Geometry: final body of the model. Coordinates: model frame, mm. Face numbers are marked on the shaded views. A direction names the side the tool comes from. Coordinates: 2 decimals unless noted, no trailing zeros. Write each loop counter-clockwise with the first axis right and the second up, starting at its lowest first coordinate (ties: lowest second). Pieces come first, ordered by that corner, then holes. Notation, with made-up numbers: (64, -5.5) -> (68, -5.5) arc R13 cw to (68, 1.5) -> close; hole circle Ø1 at (87, 82). An arc over 180 degrees is marked (long way). Answer as a JSON object with one key per item and string values. Group by question number.
```python
from build123d import *

# Parameters (mm, degrees)
SKETCH1_W           = 60
SKETCH1_H           = 30
BOSS_EXTRUDE1_DEPTH = 10
FILLET1_R           = 10
FILLET3_R           = 10
FILLET4_R           = 10
CUT_EXTRUDE1_DEPTH  = 4
CUT_EXTRUDE2_DEPTH  = 4
SKETCH8_R           = 1.5
CUT_EXTRUDE3_DEPTH  = 4
SHELL5_START        = 2
SHELL5_DEPTH        = 8
CUT_EXTRUDE4_DEPTH  = 2
SKETCH11_W          = 6.86286456
SKETCH11_H          = 3.5
BOSS_EXTRUDE2_DEPTH = 1
CUT_EXTRUDE5_DEPTH  = 0.1


# Read off the part's stored shape, not the designer's step: Shell5
with BuildPart() as part:
    # Sketch1 → Boss-Extrude1 (new body)
    with BuildSketch(Plane(origin=(0, 0, 0), x_dir=(1, 0, 0), z_dir=(0, 1, 0))):
        with Locations((-2.582747066, 7.592753862)):
            Rectangle(SKETCH1_W, SKETCH1_H)
    extrude(amount=BOSS_EXTRUDE1_DEPTH)

    # Fillet1
    fillet1_edges = [part.edges().sort_by_distance(p)[0] for p in [
        (27.417252934, 5, 7.407246138),
    ]]
    fillet(fillet1_edges, radius=FILLET1_R)

    # Fillet3
    fillet3_edges = [part.edges().sort_by_distance(p)[0] for p in [
        (-32.582747066, 5, 7.407246138),
    ]]
    fillet(fillet3_edges, radius=FILLET3_R)

    # Fillet4
    fillet4_edges = [part.edges().sort_by_distance(p)[0] for p in [
        (-32.582747066, 5, -22.592753862),
    ]]
    fillet(fillet4_edges, radius=FILLET4_R)

    # Sketch6 → Cut-Extrude1 (cut)
    with BuildSketch(Plane(origin=(0, 10, 0), x_dir=(1, 0, 0), z_dir=(0, 1, 0))):
        Polygon((17.417252934, 22.592753862), (27.417252934, 12.592753862), (27.417252934, 22.592753862), align=None)
    extrude(amount=-CUT_EXTRUDE1_DEPTH, mode=Mode.SUBTRACT)

    # Sketch7 → Cut-Extrude2 (cut)
    with BuildSketch(Plane.XZ):
        Polygon((27.417252934, -22.592753862), (27.417252934, -12.592753862), (17.417252934, -22.592753862), align=None)
    extrude(amount=-CUT_EXTRUDE2_DEPTH, mode=Mode.SUBTRACT)

    # Sketch8 → Cut-Extrude3 (cut)
    with BuildSketch(Plane(origin=(0, 6, 0), x_dir=(1, 0, 0), z_dir=(0, 1, 0))):
        with Locations(Location((24.917252934, 20.092753862, 0), (0, 0, 270))):
            Circle(SKETCH8_R)
    extrude(amount=-CUT_EXTRUDE3_DEPTH, mode=Mode.SUBTRACT)

    # Shell5 outline → Shell5 (cut)
    with BuildSketch(Plane(origin=(0, 0, 0), x_dir=(1, 0, 0), z_dir=(0, 1, 0)).offset(SHELL5_START)):
        with BuildLine():
            Line((25.417252934, 2.592753862), (25.417252934, 11.764326737))
            Line((25.417252934, 11.764326737), (16.588825809, 20.592753862))
            Line((16.588825809, 20.592753862), (-22.582747066, 20.592753862))
            ThreePointArc((-22.582747066, 20.592753862), (-28.239601315, 18.249608111), (-30.582747066, 12.592753862))
            Line((-30.582747066, 12.592753862), (-30.582747066, 2.592753862))
            ThreePointArc((-30.582747066, 2.592753862), (-28.239601315, -3.064100388), (-22.582747066, -5.407246138))
            Line((-22.582747066, -5.407246138), (17.417252934, -5.407246138))
            ThreePointArc((17.417252934, -5.407246138), (23.074107184, -3.064100387), (25.417252934, 2.592753862))
        make_face()
    extrude(amount=SHELL5_DEPTH, mode=Mode.SUBTRACT)

    # Sketch10 → Cut-Extrude4 (cut)
    with BuildSketch(Plane(origin=(0, 0, -22.592753862), x_dir=(-1, 0, 0), z_dir=(0, 0, -1))):
        Polygon((2.582747066, 5.925), (6.032747066, 5.925), (6.032747066, 4.825), (5.282747066, 4.075), (2.582747066, 4.075), (-0.117252934, 4.075), (-0.867252934, 4.825), (-0.867252934, 5.925), align=None)
    extrude(amount=-CUT_EXTRUDE4_DEPTH, mode=Mode.SUBTRACT)

    # Sketch11 → Boss-Extrude2 (add)
    with BuildSketch(Plane(origin=(0, 0, -22.592753862), x_dir=(-1, 0, 0), z_dir=(0, 0, -1))):
        with Locations((12.582747066, 5)):
            Rectangle(SKETCH11_W, SKETCH11_H)
    extrude(amount=BOSS_EXTRUDE2_DEPTH)

    # Sketch12 → Cut-Extrude5 (cut)
    with BuildSketch(Plane(origin=(0, 0, -23.592753862), x_dir=(-1, 0, 0), z_dir=(0, 0, -1))):
        Polygon((12.582747066, 5), (12.735825542, 5), (12.735825542, 6.297110067), (12.428698836, 6.297110067), (12.428698836, 5), align=None)
        with BuildLine():
            Line((12.111519237, 5.882859707), (12.204075045, 5.709453579))
            ThreePointArc((12.204075045, 5.709453579), (12.582747066, 4.195812907), (12.961419087, 5.709453579))
            Line((12.961419087, 5.709453579), (13.053974895, 5.882859707))
            ThreePointArc((13.053974895, 5.882859707), (12.582747066, 3.999251816), (12.111519237, 5.882859707))
        make_face()
    extrude(amount=-CUT_EXTRUDE5_DEPTH, mode=Mode.SUBTRACT)


solid = part.part
```
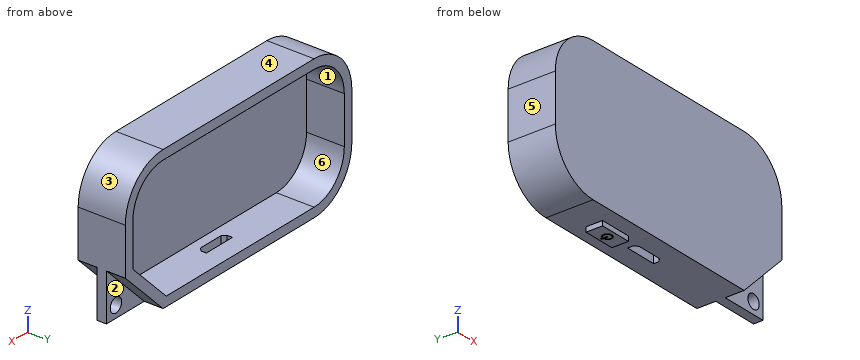
Item 1: Section A-A on y = 8.5. Output: boundary loops of the cut face in (x, z), then the cut area to 3 significant figures.
Item 2: Mould query, pull axis Z, two halves, no side actions, for the marked faces 4, 5 and 6. Classes: +Z half, -Z half, draft (parallel to the pull), parting line (faces both ways), or undercut.
Item 3: Contact query for flat-ended pins moving along their axis: pin 1 (2 mm diameter, centred on x = 7, y = 3, fed in from -Z); pin 2 (4 mm diameter, centred on x = 24.92, z = -20.09, fed in from -Y). Output: stop coordinate, or through.
Item 4: Section B-B on x = -15. Output: boundary loops of the cut face in (y, z), then the cut area to 3 significant figures.
Item 5: Section C-C on z = -20. Output: boundary loops of the cut face in (x, y).
Item 6: Ray query, L1, parallel to Z at x = -2.5, y = 4; L2, parallel to X at y = 5.75, z = -8; L3, parallel to Z at x = -11.5, y = 4.5. Return the intervals inside material, ascending. Write a range as [from, to].
Item 7: Set-up query: the marked faces 1, 2 and 3. Return all of +Z, -Z, +X, -X, +Y, -Y with unobstructed straight access to the full face (end or side cutting, diameter ignored); none if empty.
Item 8: Section D-D on y = 0.75. Output: boundary loops of the cut face in (x, z), then the cut area to 3 significant figures.
Answer sheet:
{
 "1": {"outline": "(-32.58, -12.59) arc R10 ccw to (-22.58, -22.59) -> (17.42, -22.59) -> (27.42, -12.59) -> (27.42, -2.59) arc R10 ccw to (17.42, 7.41) -> (-22.58, 7.41) arc R10 ccw to (-32.58, -2.59) -> close; hole (-30.58, -12.59) arc R8 ccw to (-22.58, -20.59) -> (16.59, -20.59) -> (25.42, -11.76) -> (25.42, -2.59) arc R8 ccw to (17.42, 5.41) -> (-22.58, 5.41) arc R8 ccw to (-30.58, -2.59) -> close", "area": "310 mm^2"},
 "2": {"face 4": "+Z half", "face 5": "draft", "face 6": "undercut"},
 "3": {"pin 1": "stops at z = -22.59", "pin 2": "stops at y = 4"},
 "4": {"outline": "(0, -22.59) -> (3.25, -22.59) -> (3.25, -23.59) -> (6.75, -23.59) -> (6.75, -22.59) -> (10, -22.59) -> (10, -20.59) -> (2, -20.59) -> (2, 5.41) -> (10, 5.41) -> (10, 7.41) -> (0, 7.41) -> close", "area": "95.5 mm^2"},
 "5": {"outline": "(-29.3, 0) -> (20.01, 0) -> (20.01, 4) -> (23.42, 4) -> (23.42, 6) -> (20.01, 6) -> (20.01, 10) -> (17.18, 10) -> (17.18, 2) -> (-25.6, 2) -> (-25.6, 10) -> (-29.3, 10) -> close; (26.41, 4) -> (27.42, 4) -> (27.42, 6) -> (26.41, 6) -> close"},
 "6": {"L1": "z = [-22.59, -20.59], [5.41, 7.41]", "L2": "x = [-32.58, -30.58], [25.42, 27.42]", "L3": "z = [-23.59, -20.59], [5.41, 7.41]"},
 "7": {"face 1": "+Y", "face 2": "-Z, +X, +Y", "face 3": "+Z, +X, +Y, -Y"},
 "8": {"outline": "(-32.58, -12.59) arc R10 ccw to (-22.58, -22.59) -> (17.42, -22.59) -> (27.42, -12.59) -> (27.42, -2.59) arc R10 ccw to (17.42, 7.41) -> (-22.58, 7.41) arc R10 ccw to (-32.58, -2.59) -> close", "area": "1,690 mm^2"}
}
